Check sheet for the modelled part. Datum: model origin and axes. Units: mm. A direction names the side the tool comes from. Give positions to 0.01 mm unless a question says otherwise; leave off trailing zeros. Write each loop counter-clockwise with the first axis right and the second up, starting at its lowest first coordinate (ties: lowest second). Pieces come first, ordered by that corner, then holes. Notation, with made-up numbers: (34, 7) -> (86, 7) arc R19 ccw to (86, 21) -> close; hole circle Ø4 at (56.5, 13.5). An arc over 180 degrees is marked (long way). Use a Markdown table: item, result. Add a question column.
1. Cross-section at A-A (x = 0.25). Enter the section's corners in (y, z) (3 decimals).
2. Cross-section at D-D (y = -1). Enter the section's corners in (x, z) (3 decimals), then the cut area to 3 significant figures.
3. Release check for a two-part mould opening along Y. For faces 1 (the cylindrical face through (-0.097, -0.781, -1.215)), 2 (the flat face through (6.95, 0, 0)), 3 (the flat face through (0, 2.75, -1)) record: released by +Y, released by -Y, zero draft, split by the parting line, or undercut.
4. Scan lines: probe 1 along Y at (x, z) = (-0.5, 0.1); probe 2 along X at (y, z) = (-1.6, -0.7); probe 3 along Y at (x, z) = (-3, -0.3). Record each from-to range of solid material in increasing order. Write a range as [from, to].
5. Cross-section at B-B (z = -0.35). Enter the section's corners in (x, y) (3 decimals), then the cut area to 3 significant figures.
6. Set-up check for faces 4 (the flat face through (0.1, 2.41, -1.475)), 5 (the flat face through (6.5, -1, -1)): record each of +Z, -Z, +X, -X, +Y, -Y from which the full face is reachable in a straight line by a thin tool's end or side.
7. Cross-section at C-C (x = -5.5). Enter the section's corners in (y, z) (3 decimals).
from build123d import *

# Parameters (mm, degrees)
SKETCH1_W               = 13
SKETCH1_H               = 4.5
BOSS_EXTRUDE1_DEPTH     = 0.225
BOSS_EXTRUDE2_DEPTH     = 1.25
BOSS_EXTRUDE3_DEPTH     = 2
SKETCH4_W               = 7
SKETCH4_H               = 0.5
CUT_EXTRUDE1_DEPTH      = 3.45
CUT_EXTRUDE2_DEPTH      = 7.95
CUT_EXTRUDE2_DEPTH_BACK = 7.95


with BuildPart() as part:
    # Sketch1 → Boss-Extrude1 (new body, symmetric)
    with BuildSketch(Plane.XY):
        Polygon((6.95, 2.25), (6.95, 2.75), (6.5, 2.75), (-6.5, 2.75), (-6.95, 2.75), (-6.95, 2.25), (-6.95, -2.25), (-6.95, -2.75), (-6.5, -2.75), (6.5, -2.75), (6.95, -2.75), (6.95, -2.25), align=None)
        Rectangle(SKETCH1_W, SKETCH1_H, mode=Mode.SUBTRACT)
        with BuildLine():
            Line((6.5, 1.875), (6.5, 2.25))
            Line((6.5, 2.25), (-6.5, 2.25))
            Line((-6.5, 2.25), (-6.5, 1.875))
            Line((-6.5, 1.875), (-6.5, 1))
            Line((-6.5, 1), (-6.5, -2.25))
            Line((-6.5, -2.25), (-2.834936491, -2.25))
            ThreePointArc((-2.834936491, -2.25), (-2.834936491, 0.25), (-5, 1.5))
            Line((-5, 1.5), (5, 1.5))
            ThreePointArc((5, 1.5), (2.834936491, 0.25), (2.834936491, -2.25))
            Line((2.834936491, -2.25), (6.5, -2.25))
            Line((6.5, -2.25), (6.5, 1))
            Line((6.5, 1), (6.5, 1.875))
        make_face()
        with BuildLine():
            Line((-2.834936491, -2.25), (2.834936491, -2.25))
            ThreePointArc((2.834936491, -2.25), (2.834936491, 0.25), (5, 1.5))
            Line((5, 1.5), (-5, 1.5))
            ThreePointArc((-5, 1.5), (-2.834936491, 0.25), (-2.834936491, -2.25))
        make_face()
    extrude(amount=BOSS_EXTRUDE1_DEPTH, both=True)

    # Sketch2 → Boss-Extrude2 (add)
    with BuildSketch(Plane(origin=(0, 0, -0.225), x_dir=(-1, 0, 0), z_dir=(0, 0, -1))):
        Polygon((-6.95, 2.25), (-6.95, -2.25), (-6.95, -2.75), (-6.5, -2.75), (6.5, -2.75), (6.95, -2.75), (6.95, -2.25), (6.95, 2.25), (6.95, 2.75), (6.5, 2.75), (-6.5, 2.75), (-6.95, 2.75), align=None)
        Polygon((-6.5, 1), (-6.5, 1.875), (-6.5, 2.25), (6.5, 2.25), (6.5, 1.875), (6.5, 1), (6.5, -2.25), (2.834936491, -2.25), (-2.834936491, -2.25), (-6.5, -2.25), align=None, mode=Mode.SUBTRACT)
    extrude(amount=BOSS_EXTRUDE2_DEPTH)

    # Sketch3 → Boss-Extrude3 (add)
    with BuildSketch(Plane(origin=(0, 0, -0.225), x_dir=(-1, 0, 0), z_dir=(0, 0, -1))):
        with BuildLine():
            ThreePointArc((-5, 1.5), (-2.834936491, 0.25), (-2.834936491, -2.25))
            Line((-2.834936491, -2.25), (2.834936491, -2.25))
            ThreePointArc((2.834936491, -2.25), (2.834936491, 0.25), (5, 1.5))
            Line((5, 1.5), (-5, 1.5))
        make_face()
    extrude(amount=BOSS_EXTRUDE3_DEPTH)

    # Sketch4 → Cut-Extrude1 (cut, through all)
    with BuildSketch(Plane(origin=(0, 0, -2.225), x_dir=(-1, 0, 0), z_dir=(0, 0, -1))):
        with Locations((0, 1.25)):
            Rectangle(SKETCH4_W, SKETCH4_H)
        with BuildLine():
            Line((3.5, 1.5), (3.5, 1))
            ThreePointArc((3.5, 1), (4.209430585, 1.371708245), (5, 1.5))
            Line((5, 1.5), (3.5, 1.5))
        make_face()
        with BuildLine():
            ThreePointArc((-5, 1.5), (-4.209430585, 1.371708245), (-3.5, 1))
            Line((-3.5, 1), (-3.5, 1.5))
            Line((-3.5, 1.5), (-5, 1.5))
        make_face()
    extrude(amount=-CUT_EXTRUDE1_DEPTH, mode=Mode.SUBTRACT)

    # Sketch5 → Cut-Extrude2 (cut, two sides)
    with BuildSketch(Plane(origin=(0, 0, 0), x_dir=(0, 0, -1), z_dir=(1, 0, 0))) as cut_extrude2_sk:
        with BuildLine():
            Line((3.725, 1.5), (0.225, 1.5))
            Line((0.225, 1.5), (0.225, 1))
            ThreePointArc((0.225, 1), (1.096708245, -1.790569415), (-1.275, -3.5))
            Line((-1.275, -3.5), (3.725, -3.5))
            Line((3.725, -3.5), (3.725, 1.5))
        make_face()
    extrude(amount=CUT_EXTRUDE2_DEPTH, mode=Mode.SUBTRACT)
    extrude(cut_extrude2_sk.sketch, amount=-CUT_EXTRUDE2_DEPTH_BACK, mode=Mode.SUBTRACT)


solid = part.part
Worked answers:
| question | item | result |
|---|---|---|
| 1 | outline | (-2.75, -0.51) arc R2.5 ccw to (1, -0.225) -> (1, 0.225) -> (-2.75, 0.225) -> close; (1.5, -0.225) -> (2.25, -0.225) -> (2.25, -1.475) -> (2.75, -1.475) -> (2.75, 0.225) -> (1.5, 0.225) -> close |
| 2 | outline | (-6.95, -1.225) -> (-6.5, -1.225) -> (-6.5, -0.225) -> (-2.5, -0.225) -> (-2.5, -1.225) -> (2.5, -1.225) -> (2.5, -0.225) -> (6.5, -0.225) -> (6.5, -1.225) -> (6.95, -1.225) -> (6.95, 0.225) -> (-6.95, 0.225) -> close |
| 2 | area | 12.2 mm² |
| 3 | face 1 | undercut |
| 3 | face 2 | zero draft |
| 3 | face 3 | released by +Y |
| 4 | probe 1 | y = [-2.75, 1], [1.5, 2.75] |
| 4 | probe 2 | x = [-6.95, -6.5], [-2.57, 2.57], [6.5, 6.95] |
| 4 | probe 3 | y = [-2.75, -2.25], [0.5, 0.94], [2.25, 2.75] |
| 5 | outline | (-6.95, -2.75) -> (6.95, -2.75) -> (6.95, 0.9) -> (6.5, 0.9) -> (6.5, -2.25) -> (2.835, -2.25) arc R2.5 cw to (3.375, 0.9) -> (-3.375, 0.9) arc R2.5 cw to (-2.835, -2.25) -> (-6.5, -2.25) -> (-6.5, 0.9) -> (-6.95, 0.9) -> close; (-6.95, 1.5) -> (-6.5, 1.5) -> (-6.5, 2.25) -> (6.5, 2.25) -> (6.5, 1.5) -> (6.95, 1.5) -> (6.95, 2.75) -> (-6.95, 2.75) -> close |
| 5 | area | 34.4 mm² |
| 6 | face 4 | -Z, +X, -X, +Y, -Y |
| 6 | face 5 | -Z |
| 7 | outline | (-2.75, -0.51) arc R2.5 ccw to (-2.25, -0.89) -> (-2.25, -0.225) -> (2.25, -0.225) -> (2.25, -1.475) -> (2.75, -1.475) -> (2.75, 0.225) -> (-2.75, 0.225) -> close |
